Check sheet for the modelled part. Datum: model origin and axes. Units: mm. Face numbers are marked on the shaded views. A direction names the side the tool comes from. Give positions to 0.01 mm unless a question says otherwise; leave off trailing zeros. Order: outer loops, then holes, each group sorted by start corner. A loop starts at its lowest first (then second) coordinate and runs counter-clockwise, first axis right, second up. Notation, with made-up numbers: (-18.75, -31.75) - (33.25, -31.75) arc R10 cw to (33.25, -27.75) - close; hole circle Ø5 at (-2, 12). An arc over 180 degrees is marked (long way). Answer in a Markdown table with one row per item.
from build123d import *

# Parameters (mm, degrees)
F2_R             = 0.2
F3_SIZE          = 2
F4_SIZE          = 1
F7_DEPTH         = 15
F7_COPIES2_COUNT = 2


# Not quite as in the source:
# - a pattern or mirror of a feature is missing from the dataset's text; its kind, count and spacing are read off the source's solid


with BuildPart() as f1:
    # F0 (on Front) → F1 (revolve)
    with BuildSketch(Plane.XZ):
        Polygon((0, 13.5), (0, 11), (22, 5), (50, 5), (50, 7.9), (25, 7.9), (25, 15), (23, 15), (23, 13.5), (15, 13.5), (15, 11.25), (11, 11.25), (11, 13.5), align=None)
    revolve(axis=Axis((18.4335876124, 0, 0), (-1, 0, 0)))

    # F2
    f2_edges = [f1.edges().sort_by_distance(p)[0] for p in [
        (50, 0, -7.9),
    ]]
    fillet(f2_edges, radius=F2_R)

    # F3
    f3_edges = [f1.edges().sort_by_distance(p)[0] for p in [
        (50, 0, -5),
        (25, 0, -7.9),
    ]]
    chamfer(f3_edges, length=F3_SIZE)

    # F4
    f4_edges = [f1.edges().sort_by_distance(p)[0] for p in [
        (0, 0, -13.5),
    ]]
    chamfer(f4_edges, length=F4_SIZE)

    # F6 (on offset) → F7 (cut)
    with BuildSketch(Plane.YZ.offset(44)):
        with BuildLine():
            ThreePointArc((-3.37, 5.4408730917), (-2.4661025438, 5.905788537), (-1.5, 6.2217360921))
            Line((-1.5, 6.2217360921), (-1.5, 7.7562877719))
            ThreePointArc((-1.5, 7.7562877719), (-2.4540983699, 7.5091544924), (-3.37, 7.145145205))
            Line((-3.37, 7.145145205), (-3.37, 5.4408730917))
        make_face()
        with BuildLine():
            Line((-5.44, 3.3714092009), (-5.44, 5.7285600285))
            ThreePointArc((-5.44, 5.7285600285), (-6.928613333, 3.7953020014), (-7.7562877719, 1.5))
            Line((-7.7562877719, 1.5), (-6.2217360921, 1.5))
            ThreePointArc((-6.2217360921, 1.5), (-5.9054690982, 2.4668673921), (-5.44, 3.3714092009))
        make_face()
    f7 = extrude(amount=-F7_DEPTH, mode=Mode.SUBTRACT)

    # F7_copies: F7 across plane
    add(f7.mirror(Plane.ZX), mode=Mode.SUBTRACT)

    # F7_copies1: F7 across plane
    add(f7.mirror(Plane(origin=(0, 0, 0), x_dir=(-1, 0, 0), z_dir=(0, 0, -1))), mode=Mode.SUBTRACT)

    # F7_copies2: F7 ×2 about axis
    f7_copies2_axis = Axis((0, 0, 0), (1, 0, 0))
    for i in range(1, F7_COPIES2_COUNT):
        add(f7.rotate(f7_copies2_axis, i * 360 / F7_COPIES2_COUNT), mode=Mode.SUBTRACT)


solid = f1.part
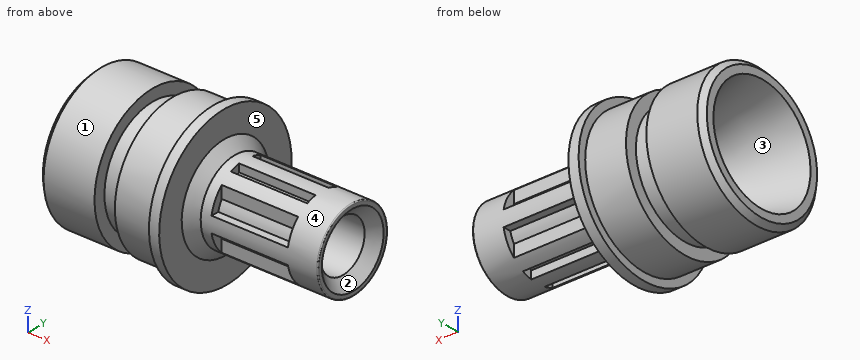
(1) Cross-section at D-D, the plane x = 12. Record the cut outline in (y, z).
Geometry says:
| item | result |
|---|---|
| outline | circle Ø22.5 at (0, 0); hole circle Ø15.45 at (0, 0) |
(2) Mould release check, pull along Y, two halves, no side actions. Record for the marked faces 3, 4 and 5: pulls with the +Y half, pulls with the -Y half, needs draft (parallel to the pull), parting line crosses it, or undercut.
Geometry says:
| item | result |
|---|---|
| face 3 | undercut |
| face 4 | parting line crosses it |
| face 5 | needs draft |
(3) Access from +Z, -Z, +X, -X, +Y, -Y to the whole of each face (thin tool, end or side, straight path). Record for the marked faces 1 and 2.
Geometry says:
| item | result |
|---|---|
| face 1 | -X |
| face 2 | +X |
(4) Gauge pin test, flat ends, axial feed: P1, Ø0.5, axis at x = 33, y = 7, coming from the -Z side; P2, Ø10, axis at x = 7, z = -1.5, coming from the +Y side; P3, Ø0.5, axis at x = 33, y = 7, coming from the +Z side. Record the tip position at first contact, or that the pin passes through.
Geometry says:
| item | result |
|---|---|
| P1 | z = -1.5 |
| P2 | y = 13.5 |
| P3 | z = 1.5 |
(5) Thickness scan on L1, parallel to Y at x = 41.75, z = 0; L2, parallel to X at y = 4.25, z = 11; L3, parallel to X at y = -6, z = -11.75. Record the ranges inside material, lowest first.
Geometry says:
| item | result |
|---|---|
| L1 | -7.9 to -5, 5 to 7.9 |
| L2 | 0 to 11, 15 to 25 |
| L3 | 0.69 to 11, 15 to 25 |
